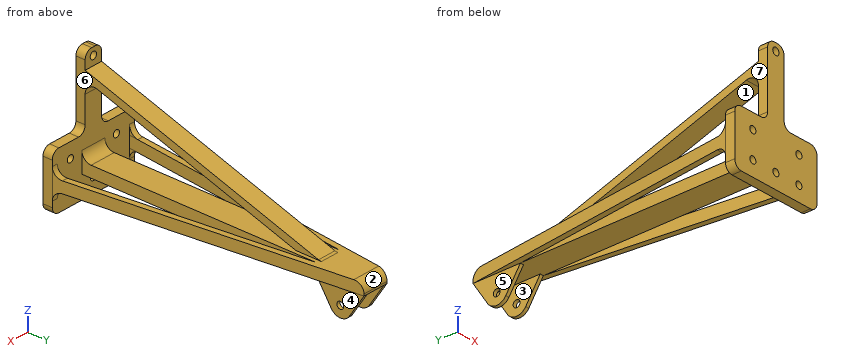
```python
from build123d import *

# Parameters (mm, degrees)
SKETCH1_W                       = 50
SKETCH1_H                       = 30
SKETCH1_R                       = 1.85
BOSS_EXTRUDE1_DEPTH             = 5
BOSS_EXTRUDE2_DEPTH             = 3
BOSS_EXTRUDE2_DEPTH_BACK        = 3
SKETCH4_R                       = 1.85
BOSS_EXTRUDE3_DEPTH             = 7
CUT_EXTRUDE1_REACH              = 162.37
SKETCH6_W                       = 10.2
SKETCH6_H                       = 14.85
SKETCH8_R                       = 1.85
SKETCH8_W                       = 10
SKETCH8_H                       = 38
SKETCH8_R_2                     = 1.917002372
BOSS_EXTRUDE4_DEPTH             = 5
BOSS_EXTRUDE5_REACH             = 169.955
BOSS_EXTRUDE5_DIRECTION_2_REACH = 169.955
FILLET1_R                       = 5
FILLET2_R                       = 4


with BuildPart() as part:
    # Sketch1 → Boss-Extrude1 (new body)
    with BuildSketch(Plane(origin=(0, 0, 0), x_dir=(1, 0, 0), z_dir=(0, 1, 0))):
        Rectangle(SKETCH1_W, SKETCH1_H)
        with Locations(Location((0, 7, 0), (0, 0, 270))):
            Circle(SKETCH1_R, mode=Mode.SUBTRACT)
        with Locations(Location((14, 7, 0), (0, 0, 270))):
            Circle(SKETCH1_R, mode=Mode.SUBTRACT)
        with Locations(Location((-14, 7, 0), (0, 0, 270))):
            Circle(SKETCH1_R, mode=Mode.SUBTRACT)
        with Locations(Location((14, -7, 0), (0, 0, 90))):
            Circle(SKETCH1_R, mode=Mode.SUBTRACT)
        with Locations(Location((0, -7, 0), (0, 0, 90))):
            Circle(SKETCH1_R, mode=Mode.SUBTRACT)
        with Locations(Location((-14, -7, 0), (0, 0, 90))):
            Circle(SKETCH1_R, mode=Mode.SUBTRACT)
    extrude(amount=BOSS_EXTRUDE1_DEPTH)

    # Sketch3 → Boss-Extrude2 (add, two sides: drawn at the far end of the back side and taken through both)
    with BuildSketch(Plane.XY.offset(-BOSS_EXTRUDE2_DEPTH_BACK)):
        Polygon((-7, 157.4), (-25, 5), (-21.97914743, 5), (-7, 131.823448239), align=None)
        Polygon((25, 5), (7, 157.4), (7, 131.823448239), (21.97914743, 5), align=None)
        Polygon((0, 157.4), (-7, 157.4), (-7, 131.823448239), (-7, 5), (0, 5), align=None)
        Polygon((7, 157.4), (0, 157.4), (0, 5), (7, 5), (7, 131.823448239), align=None)
    extrude(amount=BOSS_EXTRUDE2_DEPTH + BOSS_EXTRUDE2_DEPTH_BACK)

    # Sketch4 → Boss-Extrude3 (add)
    with BuildSketch(Plane(origin=(0, 0, 0), x_dir=(0, 0, -1), z_dir=(1, 0, 0))):
        with BuildLine():
            Line((3, 131.823448239), (15.177137146, 139.699667569))
            ThreePointArc((15.177137146, 139.699667569), (17.85, 144.611724119), (15.177137146, 149.52378067))
            Line((15.177137146, 149.52378067), (3, 157.4))
            Line((3, 157.4), (3, 131.823448239))
        make_face()
        with Locations(Location((12, 144.611724119, 0), (0, 0, 180))):
            Circle(SKETCH4_R, mode=Mode.SUBTRACT)
    boss_extrude3 = extrude(amount=BOSS_EXTRUDE3_DEPTH)

    # Mirror1: Boss-Extrude3 across plane
    add(boss_extrude3.mirror(Plane(origin=(0, 0, 0), x_dir=(0, 0, 1), z_dir=(1, 0, 0))))

    # Cut-Extrude1: up to this plane
    cut_extrude1_end = Plane(origin=(7, 91.572994836, 59.229766685), z_dir=(0, 0.8396677864426271, 0.5431003667928599))
    # Sketch6 → Cut-Extrude1 (cut, up to the surface)
    with BuildSketch(Plane(origin=(0, 157.4, 0), x_dir=(1, 0, 0), z_dir=(0, 1, 0)), mode=Mode.PRIVATE) as cut_extrude1_sk1:
        with Locations((0, 10.425)):
            Rectangle(SKETCH6_W, SKETCH6_H)
    cut_extrude1_tool1 = split(extrude(cut_extrude1_sk1.sketch, amount=-CUT_EXTRUDE1_REACH, mode=Mode.PRIVATE), bisect_by=cut_extrude1_end, keep=Keep.BOTH, mode=Mode.PRIVATE)
    add(cut_extrude1_tool1.solids().sort_by_distance((0, 157.4, -10.425))[0], mode=Mode.SUBTRACT)

    # Sketch8 → Boss-Extrude4 (add)
    # profile 1 of 2: a face of its own
    with BuildSketch(Plane.XZ):
        with Locations((0, 7)):
            Circle(SKETCH8_R)
    # profile 2 of 2: a face of its own
    with BuildSketch(Plane.XZ):
        with Locations((0, 34)):
            Rectangle(SKETCH8_W, SKETCH8_H)
        with Locations(Location((0, 49, 0), (0, 0, 270))):
            Circle(SKETCH8_R_2, mode=Mode.SUBTRACT)
    extrude(amount=-BOSS_EXTRUDE4_DEPTH)

    # Boss-Extrude5: up to this face of the body (flat: up to its plane)
    boss_extrude5_end = Plane(part.part.faces().sort_by_distance((5, 2.5, 34))[0])
    # Sketch9 → Boss-Extrude5 (add, up to the picked face)
    with BuildSketch(Plane(origin=(0, 0, 0), x_dir=(0, 0, -1), z_dir=(1, 0, 0)), mode=Mode.PRIVATE) as boss_extrude5_sk1:
        Polygon((-3, 131.823448239), (-44.205833274, 5), (-40, 5), (-3, 118.878720851), align=None)
    boss_extrude5_tool1 = split(extrude(boss_extrude5_sk1.sketch, amount=BOSS_EXTRUDE5_REACH, mode=Mode.PRIVATE), bisect_by=boss_extrude5_end, keep=Keep.BOTH, mode=Mode.PRIVATE)
    add(boss_extrude5_tool1.solids().sort_by(Axis((0, 65.233555, 22.570307), (1, 0, 0)))[0])

    # Boss-Extrude5 direction 2: up to this face of the body (flat: up to its plane)
    boss_extrude5_direction_2_end = Plane(part.part.faces().sort_by_distance((-5, 2.5, 34))[0])
    # Sketch9 → Boss-Extrude5 direction 2 (add, up to the picked face)
    with BuildSketch(Plane(origin=(0, 0, 0), x_dir=(0, 0, -1), z_dir=(1, 0, 0)), mode=Mode.PRIVATE) as boss_extrude5_direction_2_sk1:
        Polygon((-3, 131.823448239), (-44.205833274, 5), (-40, 5), (-3, 118.878720851), align=None)
    boss_extrude5_direction_2_tool1 = split(extrude(boss_extrude5_direction_2_sk1.sketch, amount=-BOSS_EXTRUDE5_DIRECTION_2_REACH, mode=Mode.PRIVATE), bisect_by=boss_extrude5_direction_2_end, keep=Keep.BOTH, mode=Mode.PRIVATE)
    add(boss_extrude5_direction_2_tool1.solids().sort_by(Axis((0, 65.233555, 22.570307), (-1, 0, 0)))[0])

    # Fillet1
    # the kernel refuses this fillet: 5 mm, written as the material it adds along each edge
    with BuildSketch(Plane(origin=(-5, 131.823448239, 3), x_dir=(0, -0.9510600491338266, 0.3090061212040359), z_dir=(1, 0, 0))) as fillet1_piece_1:
        with BuildLine():
            CenterArc((FILLET1_R * 0.158378580578, -FILLET1_R), FILLET1_R, 90, 17.999344954)
            Line((-FILLET1_R * 0.150627540626, -FILLET1_R * 0.0489399508662), (0, 0))
            Line((0, 0), (FILLET1_R * 0.158378580578, 0))
        make_face()
    extrude(amount=10)
    with BuildSketch(Plane(origin=(-5, 5, 40), x_dir=(0, 0.9510600491338281, -0.3090061212040312), z_dir=(1, 0, 0))) as fillet1_piece_2:
        with BuildLine():
            CenterArc((FILLET1_R * 1.37636537503, -FILLET1_R), FILLET1_R, 90, 107.999344954)
            Line((FILLET1_R * 0.425305325898, -FILLET1_R * 1.3090061212), (0, 0))
            Line((0, 0), (FILLET1_R * 1.37636537503, 0))
        make_face()
    extrude(amount=10)
    with BuildSketch(Plane(origin=(9.47914743, 5, 3), x_dir=(0, 1, 0), z_dir=(1, 0, 0))) as fillet1_piece_3_section:
        with BuildLine():
            CenterArc((FILLET1_R, FILLET1_R), FILLET1_R, 180, 90)
            Line((0, FILLET1_R), (0, 0))
            Line((0, 0), (FILLET1_R, 0))
        make_face()
    fillet1_piece_3 = extrude(amount=15.52085257, mode=Mode.PRIVATE)
    fillet1_piece_3 = split(fillet1_piece_3, bisect_by=Plane(origin=(21.86620474, 5.956248104, 4.13176941), z_dir=(0.9930971241558421, 0.11729493592391835, 0)), keep=Keep.TOP, mode=Mode.PRIVATE)
    fillet1_piece_3 = split(fillet1_piece_3, bisect_by=Plane(origin=(24.845496113, 6.308132911, 4.13176941), z_dir=(-0.9930971241558421, -0.11729493592391835, 0)), keep=Keep.TOP, mode=Mode.PRIVATE)
    add(fillet1_piece_3)
    with BuildSketch(Plane(origin=(-25, 5, -3), x_dir=(0, 1, 0), z_dir=(1, 0, 0))) as fillet1_piece_4_section:
        with BuildLine():
            CenterArc((FILLET1_R, -FILLET1_R), FILLET1_R, 90, 90)
            Line((0, -FILLET1_R), (0, 0))
            Line((0, 0), (FILLET1_R, 0))
        make_face()
    fillet1_piece_4 = extrude(amount=15.52085257, mode=Mode.PRIVATE)
    fillet1_piece_4 = split(fillet1_piece_4, bisect_by=Plane(origin=(-24.845496113, 6.308132911, -4.13176941), z_dir=(0.9930971241558421, -0.11729493592391835, 0)), keep=Keep.TOP, mode=Mode.PRIVATE)
    fillet1_piece_4 = split(fillet1_piece_4, bisect_by=Plane(origin=(-21.86620474, 5.956248104, -4.13176941), z_dir=(-0.9930971241558421, 0.11729493592391835, 0)), keep=Keep.TOP, mode=Mode.PRIVATE)
    add(fillet1_piece_4)
    with BuildSketch(Plane(origin=(9.47914743, 5, -3), x_dir=(0, 1, 0), z_dir=(1, 0, 0))) as fillet1_piece_5_section:
        with BuildLine():
            CenterArc((FILLET1_R, -FILLET1_R), FILLET1_R, 90, 90)
            Line((0, -FILLET1_R), (0, 0))
            Line((0, 0), (FILLET1_R, 0))
        make_face()
    fillet1_piece_5 = extrude(amount=15.52085257, mode=Mode.PRIVATE)
    fillet1_piece_5 = split(fillet1_piece_5, bisect_by=Plane(origin=(24.845496113, 6.308132911, -4.13176941), z_dir=(-0.9930971241558421, -0.11729493592391835, 0)), keep=Keep.TOP, mode=Mode.PRIVATE)
    fillet1_piece_5 = split(fillet1_piece_5, bisect_by=Plane(origin=(21.86620474, 5.956248104, -4.13176941), z_dir=(0.9930971241558421, 0.11729493592391835, 0)), keep=Keep.TOP, mode=Mode.PRIVATE)
    add(fillet1_piece_5)
    with BuildSketch(Plane(origin=(-25, 5, 3), x_dir=(0, 1, 0), z_dir=(1, 0, 0))) as fillet1_piece_6_section:
        with BuildLine():
            CenterArc((FILLET1_R, FILLET1_R), FILLET1_R, 180, 90)
            Line((0, FILLET1_R), (0, 0))
            Line((0, 0), (FILLET1_R, 0))
        make_face()
    fillet1_piece_6 = extrude(amount=15.52085257, mode=Mode.PRIVATE)
    fillet1_piece_6 = split(fillet1_piece_6, bisect_by=Plane(origin=(-24.845496113, 6.308132911, 4.13176941), z_dir=(0.9930971241558421, -0.11729493592391835, 0)), keep=Keep.TOP, mode=Mode.PRIVATE)
    fillet1_piece_6 = split(fillet1_piece_6, bisect_by=Plane(origin=(-21.86620474, 5.956248104, 4.13176941), z_dir=(-0.9930971241558421, 0.11729493592391835, 0)), keep=Keep.TOP, mode=Mode.PRIVATE)
    add(fillet1_piece_6)
    with BuildSketch(Plane(origin=(-7, 5, 3), x_dir=(0, 1, 0), z_dir=(1, 0, 0))) as fillet1_piece_7:
        with BuildLine():
            CenterArc((FILLET1_R, FILLET1_R), FILLET1_R, 180, 90)
            Line((0, FILLET1_R), (0, 0))
            Line((0, 0), (FILLET1_R, 0))
        make_face()
    extrude(amount=14)
    # the kernel refuses this fillet: 5 mm, written as the material it takes off along each edge
    with BuildSketch(Plane(origin=(-19.5, 157.4, 3), x_dir=(0, -1, 0), z_dir=(1, 0, 0))) as fillet1_2_piece_1:
        with BuildLine():
            CenterArc((FILLET1_R, FILLET1_R), FILLET1_R, 180, 90)
            Line((0, FILLET1_R), (0, 0))
            Line((0, 0), (FILLET1_R, 0))
        make_face()
    extrude(amount=39, mode=Mode.SUBTRACT)

    # Fillet2
    fillet2_edges = [part.edges().sort_by_distance(p)[0] for p in [
        (5, 2.5, 15),
        (5, 2.5, 53),
        (-5, 2.5, 53),
        (-5, 2.5, 15),
        (25, 2.5, 15),
        (-25, 2.5, 15),
        (-25, 2.5, -15),
        (25, 2.5, -15),
    ]]
    fillet(fillet2_edges, radius=FILLET2_R)


solid = part.part
```
Geometry: final body of the model. Coordinates: model frame, mm. Face numbers are marked on the shaded views. A direction names the side the tool comes from. Coordinates: 2 decimals unless noted, no trailing zeros. Order: outer loops, then holes, each group sorted by start corner. A loop starts at its lowest first (then second) coordinate and runs counter-clockwise, first axis right, second up. Notation, with made-up numbers: (8.25, 63) -> (30.25, 63) arc R25 cw to (30.25, 81) -> close; hole circle Ø9 at (39, -26). An arc over 180 degrees is marked (long way). Write each question's results on one line, items separated by ' | '. Start each with the question number.
1) First-contact query: pin 1 (24 mm diameter, centred on x = -6.5, z = 14.5, fed in from +Y); pin 2 (2 mm diameter, centred on x = 7, y = 66, fed in from +Z); pin 3 (12 mm diameter, centred on x = -10.5, y = 110.5, fed in from -Z). Flat tips, straight axial feed; report the tip coordinate or a pass-through.
2) Material intervals for line 1 along X through (y, z) = (3.8, -7); line 2 along X through (y, z) = (3, 7); line 3 along Y through (x, z) = (6, -12), sorted ascending.
3) Cut plane B-B, the plane z = 21. Output: boundary loops of the cut face in (x, y).
4) Mould query, pull axis Z, two halves, no side actions, for the marked faces 1, 2 and 3. Classes: released by +Z, released by -Z, zero draft, split by the parting line, or undercut.
5) Set-up query: the marked faces 4, 5, 6 and 7. Return all of +Z, -Z, +X, -X, +Y, -Y with unobstructed straight access to the full face (end or side cutting, diameter ignored); none if empty.
6) Cut plane C-C, the plane x = -14. Output: boundary loops of the cut face in (y, z).
7) Cut plane D-D, the plane y = 129. Output: boundary loops of the cut face in (x, z), and give its area (3 significant figures).
8) Cut plane A-A, the plane y = 113. Output: boundary loops of the cut face in (x, z).
Checks:
1) pin 1: y = 154.58 | pin 2: z = 3 | pin 3: z = -3
2) line 1: -25 to -15.85, -12.15 to -1.85, 1.85 to 12.15, 15.85 to 25 | line 2: -25 to -15.85, -12.15 to 12.15, 15.85 to 25 | line 3: 0 to 5, 137.64 to 142.76, 146.46 to 151.58
3) outline: (-5, 0) -> (5, 0) -> (5, 5) -> (-5, 5) -> close; (-5, 63.48) -> (5, 63.48) -> (5, 76.42) -> (-5, 76.42) -> close
4) face 1: undercut | face 2: released by +Z | face 3: zero draft
5) face 4: -Z, +X, +Y | face 5: -Z, -X, +Y | face 6: +Z, +X, +Y | face 7: +Z, -X, +Y
6) outline: (0, -15) -> (5, -15) -> (5, -8.85) -> (0, -8.85) -> close; (0, -5.15) -> (5, -5.15) -> (5, 5.15) -> (0, 5.15) -> close; (0, 8.85) -> (5, 8.85) -> (5, 15) -> (0, 15) -> close; (72.56, -3) -> (98.13, -3) -> (98.13, 3) -> (72.56, 3) -> close
7) outline: (-10.35, -3) -> (-7.33, -3) -> (-7.33, 3) -> (-10.35, 3) -> close; (-7, -3) -> (7, -3) -> (7, 3) -> (5, 3) -> (5, 3.92) -> (-5, 3.92) -> (-5, 3) -> (-7, 3) -> close; (7.33, -3) -> (10.35, -3) -> (10.35, 3) -> (7.33, 3) -> close | area: 129 mm^2
8) outline: (-12.24, -3) -> (-9.22, -3) -> (-9.22, 3) -> (-12.24, 3) -> close; (-7, -3) -> (7, -3) -> (7, 3) -> (-7, 3) -> close; (-5, 4.91) -> (5, 4.91) -> (5, 9.12) -> (-5, 9.12) -> close; (9.22, -3) -> (12.24, -3) -> (12.24, 3) -> (9.22, 3) -> close
